```python
from build123d import *

# Parameters (mm, degrees)
F2_R     = 5.55625
F5_R     = 8.5725
F6_DEPTH = 4.7625
F8_R     = 5.55625
F9_DEPTH = 38.1


with BuildPart() as f3:
    # F3: sweep along a path in F0
    with BuildLine(Plane.XY) as f3_path:
        Line((-11.90625, -24.6450335324), (-11.90625, -21.4642974367))
        ThreePointArc((-11.90625, -21.4642974367), (-12.4922697511, -18.7998966242), (-14.142165493, -16.6272726623))
        ThreePointArc((-14.142165493, -16.6272726623), (0, 21.828125), (14.142165493, -16.6272726623))
        ThreePointArc((14.142165493, -16.6272726623), (12.4922697511, -18.7998966242), (11.90625, -21.4642974367))
        Line((11.90625, -21.4642974367), (11.90625, -24.6450335324))
    # F2 (on line) → F3 (sweep)
    with BuildSketch(Plane(origin=(0, -24.6450335324, 0), x_dir=(-1, 0, 0), z_dir=(0, 1, 0))):
        with Locations((11.90625, 0)):
            Circle(F2_R)
    sweep(path=f3_path.line)

    # F5 (on plane+point) → F6 (join, symmetric)
    with BuildSketch(Plane.YZ.offset(-11.90625)):
        with Locations((-30.9950335324, 0)):
            Circle(F5_R)
    extrude(amount=F6_DEPTH, both=True)

    # F7: F3 across plane


with BuildPart() as f3_1:
    add(f3.part)
    add(f3.part.mirror(Plane.YZ))

    # F8 (on face) → F9 (join)
    with BuildSketch(Plane(origin=(-16.66875, 0, 0), x_dir=(0, -1, 0), z_dir=(-1, 0, 0))):
        with Locations((30.9950335324, 0)):
            Circle(F8_R)
    extrude(amount=-F9_DEPTH)


solid = f3_1.part
```
Read the model definition and answer for the solid it produces. Units are mm, in the model's axes. A direction names the side the tool comes from. Coordinates: 2 decimals unless noted, no trailing zeros. Write each loop counter-clockwise with the first axis right and the second up, starting at its lowest first coordinate (ties: lowest second). Pieces come first, ordered by that corner, then holes. Notation, with made-up numbers: (81.5, -3.75) -> (107.5, -3.75) arc R20 ccw to (107.5, 32.25) -> close; hole circle Ø3 at (89.25, 89). An arc over 180 degrees is marked (long way). Return JSON: item names as keys, results as strings.
1. Find the intervals of material crossed by line 1 along X through (y, z) = (-27, 4.25); line 2 along X through (y, z) = (-7, 4.25); line 3 along Y through (x, z) = (1, 0.5), in increasing order. Write a range as from..to.
Found:
{"line 1": "-16.67..-7.14, 7.14..16.67", "line 2": "-24.42..-16.85, 16.85..24.42", "line 3": "-36.53..-25.46, 16.26..27.34"}
2. Each of these flat-tipped pins is pushed along its axis until it touches: P1, Ø8, axis at x = -9.5, z = 6.5, coming from the -Y side; P2, Ø5, axis at y = -34.5, z = 1.5, coming from the +X side; P3, Ø0.9, axis at x = -17, z = 0, coming from the -Y side; P4, Ø10, axis at x = 17.5, y = -22.5, coming from the +Z side. Where does it stop, or does it pass through?
Found:
{"P1": "y = -39.19", "P2": "x = 21.43", "P3": "y = -39.57", "P4": "z = 7.8"}
3. A cutting plane is placed at B-B (z = 1.5). Determine the outline of the cut face in (x, y), and give its area (3 significant figures).
Found:
{"outline": "(-17.61, -20.7) arc R1 cw to (-17.26, -21.46) -> (-17.26, -24.65) -> (-16.67, -24.65) -> (-16.67, -39.44) -> (-7.14, -39.44) -> (-7.14, -36.34) -> (7.14, -36.34) -> (7.14, -39.44) -> (16.67, -39.44) -> (16.67, -36.34) -> (21.43, -36.34) -> (21.43, -25.65) -> (16.67, -25.65) -> (16.67, -24.65) -> (17.26, -24.65) -> (17.26, -21.46) arc R1 cw to (17.61, -20.7) arc R27.18 ccw (long way) to start; hole (-10.68, -12.55) arc R11.7 cw to (-6.56, -21.46) -> (-6.56, -24.65) -> (-7.14, -24.65) -> (-7.14, -25.65) -> (7.14, -25.65) -> (7.14, -24.65) -> (6.56, -24.65) -> (6.56, -21.46) arc R11.7 cw to (10.68, -12.55) arc R16.48 ccw (long way) to start", "area": "1,810 mm2"}
4. A cutting plane is placed at A-A (z = -4.5). Determine the outline of the cut face in (x, y).
Found:
{"outline": "(-16.67, -38.29) -> (-7.14, -38.29) -> (-7.14, -34.25) -> (7.14, -34.25) -> (7.14, -38.29) -> (16.67, -38.29) -> (16.67, -34.25) -> (21.43, -34.25) -> (21.43, -27.74) -> (16.67, -27.74) -> (16.67, -23.7) -> (15.17, -23.7) -> (15.17, -21.46) arc R3.09 cw to (16.25, -19.11) arc R25.09 ccw (long way) to (-16.25, -19.11) arc R3.09 cw to (-15.17, -21.46) -> (-15.17, -23.7) -> (-16.67, -23.7) -> close; hole (-12.03, -14.14) arc R9.61 cw to (-8.65, -21.46) -> (-8.65, -23.7) -> (-7.14, -23.7) -> (-7.14, -27.74) -> (7.14, -27.74) -> (7.14, -23.7) -> (8.65, -23.7) -> (8.65, -21.46) arc R9.61 cw to (12.03, -14.14) arc R18.57 ccw (long way) to start"}
5. A tool of negligible diameter and unlimited length cuts with its end or side. For faces 4 (the face through (19.017, -25.444, 0.244)), 5 (the face through (7.144, -37, 0)), from which of +Z, -Z, +X, -X, +Y, -Y can it reach the whole face along a straight path? Write none if from no direction.
Found:
{"face 4": "+X", "face 5": "none"}
6. Determine the mould class of faces 1 (the face through (16.669, -37, 0)), 2 (the face through (21.431, -31, 0)), 3 (the face through (17.04, -22.72, -2.13)) for opening direction Y: pulls with the +Y half, pulls with the -Y half, needs draft (parallel to the pull), parting line crosses it, or undercut.
Found:
{"face 1": "undercut", "face 2": "needs draft", "face 3": "undercut"}
